Verification items for the finished model (mm, model axes). A direction names the side the tool comes from. Give positions to 0.01 mm unless a question says otherwise; leave off trailing zeros. Write each loop counter-clockwise with the first axis right and the second up, starting at its lowest first coordinate (ties: lowest second). Pieces come first, ordered by that corner, then holes. Notation, with made-up numbers: (-19, 6.5) -> (-12, 6.5) arc R36 ccw to (-12, 44.5) -> close; hole circle Ø3 at (-5, 44). An arc over 180 degrees is marked (long way). Use one line per item in the form item = value. Start each with the question number.
(1) Depth check by flat-ended pin: pin 1 Ø3 at (x, z) = (-2.5, 2.5) entering from +Y; pin 2 Ø3 at (x, y) = (-52, -14.5) entering from +Z; pin 3 Ø2.5 at (y, z) = (2.5, 26) entering from +X. Enter the tip coordinate at first touch or a pass-through.
(2) Set-up check for faces 1 (the face through (-5.25, 2, 41)), 2 (the face through (48, 0, 108)), 3 (the face through (0, 0, 38)), 4 (the face through (0, 5, 38)): record each of +Z, -Z, +X, -X, +Y, -Y from which the full face is reachable in a straight line by a thin tool's end or side.
(3) Scan lines: L1, parallel to X at y = 1.75, z = 2.5; L2, parallel to Z at x = 20, y = -8.5; L3, parallel to Y at x = 67, z = 90. Record each from-to range of solid material in increasing order.
(4) Section check A-A, the plane x = 42. Record the cut outline in (y, z).
(5) Release check for a two-part mould opening along Z. For faces 5 (the face through (0.3, 21, 109.5)), 6 (the face through (-1, 0, 108.5)), 7 (the face through (0.1, 2.5, -10.5)) record: pulls with the +Z half, pulls with the -Z half, needs draft (parallel to the pull), parting line crosses it, or undercut.
(6) Section check B-B, the plane z = 86. Record the cut outline in (x, y).
from build123d import *

# Parameters (mm, degrees)
SKETCH1_R               = 1.4
BOSS_EXTRUDE1_DEPTH     = 5
SKETCH3_W               = 139.5
SKETCH3_H               = 50
SKETCH3_R               = 1.4
BOSS_EXTRUDE3_DEPTH     = 5
CUT_EXTRUDE1_DEPTH      = 136.544503915
CUT_EXTRUDE1_DEPTH_BACK = 136.544503915
FILLET1_START           = -25
FILLET1_DEPTH           = 50
FILLET1_START_2         = -21.62169291
FILLET1_2_DEPTH         = 43.24338582
FILLET1_START_3         = -69.75
FILLET1_3_DEPTH         = 139.5


with BuildPart() as part:
    # Sketch1 → Boss-Extrude1 (new body)
    with BuildSketch(Plane(origin=(0, 0, 0), x_dir=(1, 0, 0), z_dir=(0, 1, 0))):
        with BuildLine():
            Line((-5.25, 5.25), (-5.25, -88.5))
            Line((-5.25, -88.5), (5.25, -88.5))
            Line((5.25, -88.5), (5.25, 5.25))
            ThreePointArc((5.25, 5.25), (0, 10.5), (-5.25, 5.25))
        make_face()
        with Locations(Location((-2.5, 2.5, 0), (0, 0, 270))):
            Circle(SKETCH1_R, mode=Mode.SUBTRACT)
        with Locations(Location((2.5, 2.5, 0), (0, 0, 90))):
            Circle(SKETCH1_R, mode=Mode.SUBTRACT)
        with Locations(Location((-2.5, -2.5, 0), (0, 0, 90))):
            Circle(SKETCH1_R, mode=Mode.SUBTRACT)
        with Locations(Location((2.5, -2.5, 0), (0, 0, 270))):
            Circle(SKETCH1_R, mode=Mode.SUBTRACT)
    extrude(amount=BOSS_EXTRUDE1_DEPTH)

    # Sketch3 → Boss-Extrude3 (add)
    with BuildSketch(Plane.XY.offset(88.5)):
        Rectangle(SKETCH3_W, SKETCH3_H)
        with Locations((-67, 0)):
            Circle(SKETCH3_R, mode=Mode.SUBTRACT)
        with Locations(Location((67, 0, 0), (0, 0, 180))):
            Circle(SKETCH3_R, mode=Mode.SUBTRACT)
    extrude(amount=BOSS_EXTRUDE3_DEPTH)

    # Sketch4 → Loft1 section 0
    with BuildSketch(Plane.XY.offset(93.5)):
        with BuildLine():
            Line((69.75, -25), (69.75, 25))
            Line((69.75, 25), (-69.75, 25))
            Line((-69.75, 25), (-69.75, -25))
            Line((-69.75, -25), (69.75, -25))
        make_face()
    # Sketch5 → Loft1 section 1
    with BuildSketch(Plane.XY.offset(113.5)):
        with BuildLine():
            Line((-50, -20), (50, -20))
            Line((50, -20), (50, 20))
            Line((50, 20), (-50, 20))
            Line((-50, 20), (-50, -20))
        make_face()
    loft()

    # Sketch6 → Cut-Extrude1 (cut, two sides: drawn at the far end of the back side and taken through both)
    with BuildSketch(Plane(origin=(0, 0, 0), x_dir=(1, 0, 0), z_dir=(0, 1, 0)).offset(-CUT_EXTRUDE1_DEPTH_BACK)):
        Polygon((-47.910487388, -108.5), (47.910487388, -108.5), (62.722987388, -93.5), (-62.722987388, -93.5), align=None)
    extrude(amount=CUT_EXTRUDE1_DEPTH + CUT_EXTRUDE1_DEPTH_BACK, mode=Mode.SUBTRACT)

    # Fillet1: read off the stored shape, not the designer's step
    # Fillet1 outline → Fillet1 (add)
    with BuildSketch(Plane(origin=(0, 0, 0), x_dir=(1, 0, 0), z_dir=(0, 1, 0)).offset(FILLET1_START)):
        with BuildLine():
            Line((-62.722987388, -93.5), (-54.316174382, -102.013228361))
            ThreePointArc((-54.316174382, -102.013228361), (-55.371832653, -96.572066106), (-50.758474776, -93.5))
            Line((-50.758474776, -93.5), (-62.722987388, -93.5))
        make_face()
        with BuildLine():
            ThreePointArc((50.758474776, -93.5), (55.371832653, -96.572066106), (54.316174382, -102.013228361))
            Line((54.316174382, -102.013228361), (62.722987388, -93.5))
            Line((62.722987388, -93.5), (50.758474776, -93.5))
        make_face()
    extrude(amount=FILLET1_DEPTH)

    # Fillet1 2 outline → Fillet1 2 (add)
    with BuildSketch(Plane(origin=(0, 0, 0), x_dir=(1, 0, 0), z_dir=(0, 1, 0)).offset(FILLET1_START_2)):
        with BuildLine():
            Line((-47.910487388, -108.5), (-45.820974776, -108.5))
            ThreePointArc((-45.820974776, -108.5), (-47.74890867, -108.113357877), (-49.378674382, -107.013228361))
            Line((-49.378674382, -107.013228361), (-47.910487388, -108.5))
        make_face()
        with BuildLine():
            ThreePointArc((49.378674382, -107.013228361), (47.74890867, -108.113357877), (45.820974776, -108.5))
            Line((45.820974776, -108.5), (47.910487388, -108.5))
            Line((47.910487388, -108.5), (49.378674382, -107.013228361))
        make_face()
    extrude(amount=FILLET1_2_DEPTH)

    # Fillet1 3 outline → Fillet1 3 (cut)
    with BuildSketch(Plane.YZ.offset(FILLET1_START_3)):
        Polygon((25, 93.5), (25, 110), (20.875, 110), align=None)
        Polygon((-20.875, 110), (-25, 110), (-25, 93.5), align=None)
    extrude(amount=FILLET1_3_DEPTH, mode=Mode.SUBTRACT)


solid = part.part
Completed:
q1.pin_1 = 5
q1.pin_2 = 112.99
q1.pin_3 = 5.25
q2.face_1 = -Z, -X, +Y, -Y
q2.face_2 = +Y, -Y
q2.face_3 = -Z, +X, -X, -Y
q2.face_4 = -Z, +X, -X, +Y
q3.L1 = -5.25 to -3.9, -1.1 to 1.1, 3.9 to 5.25
q3.L2 = 88.5 to 93.5, 108.5 to 113.5
q3.L3 = -25 to -1.4, 1.4 to 25
q4.outline = (-25, 88.5) -> (25, 88.5) -> (25, 93.5) -> (-25, 93.5) -> close; (-21.25, 108.5) -> (21.25, 108.5) -> (20, 113.5) -> (-20, 113.5) -> close
q5.face_5 = pulls with the +Z half
q5.face_6 = undercut
q5.face_7 = pulls with the -Z half
q6.outline = (-5.25, 0) -> (5.25, 0) -> (5.25, 5) -> (-5.25, 5) -> close
